Read the model definition and answer for the solid it produces. Units are mm, in the model's axes. Face numbers are marked on the shaded views. A direction names the side the tool comes from. Coordinates: 2 decimals unless noted, no trailing zeros. Loops run counter-clockwise (first coordinate to the right, second up) from the corner with the lowest first, then second, coordinate; pieces in that order, holes last. Notation, with made-up numbers: (38.25, 1.5) - (74.25, 1.5) arc R13 cw to (74.25, 13.5) - close; hole circle Ø7 at (-28.5, 2). An arc over 180 degrees is marked (long way). Use one line per item in the form item = value.
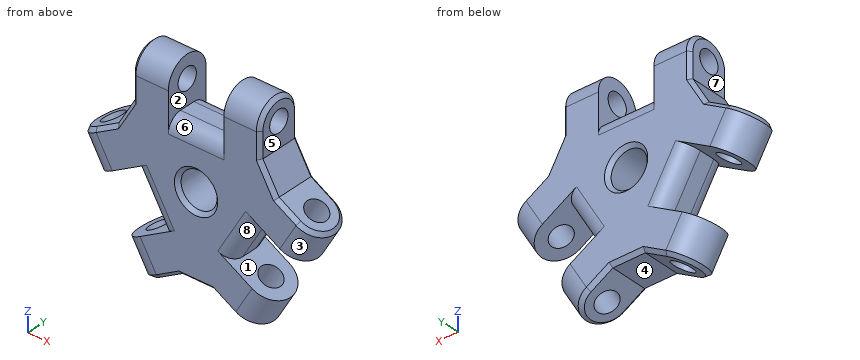
from build123d import *

# Parameters (mm, degrees)
SKETCH1_R           = 2.5
BOSS_EXTRUDE1_DEPTH = 3.1
CUT_EXTRUDE1_START  = -26.968876556
SKETCH2_R           = 1.5
CUT_EXTRUDE1_DEPTH  = 36.237753113
CIRPATTERN5_COUNT   = 3
FILLET2_R           = 2
CHAMFER1_SIZE       = 0.5


with BuildPart() as part:
    # Sketch1 → Boss-Extrude1 (new body, symmetric)
    with BuildSketch(Plane(origin=(0, 0, 0), x_dir=(1, 0, 0), z_dir=(0, 1, 0))):
        Polygon((-8.85, -7.707626094), (-8.85, -14.657626094), (-3.85, -14.657626094), (-3.85, -7.707626094), (3.85, -7.707626094), (3.85, -14.657626094), (8.85, -14.657626094), (8.85, -7.707626094), (11.1, -3.810511777), (17.118876556, -0.335511777), (14.618876556, 3.994615242), (8.6, 0.519615242), (4.75, 7.188010851), (10.768876556, 10.663010851), (8.268876556, 14.99313787), (2.25, 11.51813787), (-2.25, 11.51813787), (-8.268876556, 14.99313787), (-10.768876556, 10.663010851), (-4.75, 7.188010851), (-8.6, 0.519615242), (-14.618876556, 3.994615242), (-17.118876556, -0.335511777), (-11.1, -3.810511777), align=None)
        Circle(SKETCH1_R, mode=Mode.SUBTRACT)
    extrude(amount=BOSS_EXTRUDE1_DEPTH, both=True)

    # Sketch2 → Cut-Extrude1 (cut)
    with BuildSketch(Plane.ZY.offset(8.85).offset(CUT_EXTRUDE1_START)):
        with Locations((11.182626094, 0)):
            Circle(SKETCH2_R)
        with BuildLine():
            Line((11.182626094, 3.1), (14.657626094, 3.1))
            Line((14.657626094, 3.1), (14.657626094, -3.1))
            Line((14.657626094, -3.1), (11.182626094, -3.1))
            ThreePointArc((11.182626094, -3.1), (14.282626094, 0), (11.182626094, 3.1))
        make_face()
    cut_extrude1 = extrude(amount=CUT_EXTRUDE1_DEPTH, mode=Mode.SUBTRACT)

    # CirPattern5: Cut-Extrude1 ×3 about axis
    cirpattern5_axis = Axis((0, 3.1, 0), (0, -1, 0))
    for i in range(1, CIRPATTERN5_COUNT):
        add(cut_extrude1.rotate(cirpattern5_axis, i * 360 / CIRPATTERN5_COUNT), mode=Mode.SUBTRACT)

    # Fillet2
    fillet2_edges = [part.edges().sort_by_distance(p)[0] for p in [
        (6.675, 3.1, -3.853813047),
        (0, -3.1, 7.707626094),
        (-6.675, -3.1, -3.853813047),
        (6.675, -3.1, -3.853813047),
        (-6.675, 3.1, -3.853813047),
        (0, 3.1, 7.707626094),
    ]]
    fillet(fillet2_edges, radius=FILLET2_R)

    # Chamfer1
    chamfer1_edges = [part.edges().sort_by_distance(p)[0] for p in [
        (-12.604719139, -3.1, 2.941761777),
        (-12.604719139, 3.1, 2.941761777),
        (-16.79411703, 0, 0.523011777),
        (3.754719139, -3.1, -12.38688787),
        (3.754719139, 3.1, -12.38688787),
        (7.94411703, 0, -14.80563787),
        (16.79411703, 0, 0.523011777),
        (-7.94411703, 0, -14.80563787),
        (-8.85, -3.1, 9.445126094),
        (-9.975, -3.1, 5.759068935),
        (-3.754719139, -3.1, -12.38688787),
        (0, -3.1, -11.51813787),
        (12.604719139, -3.1, 2.941761777),
        (9.975, -3.1, 5.759068935),
        (0, 3.1, -11.51813787),
        (-3.754719139, 3.1, -12.38688787),
        (9.975, 3.1, 5.759068935),
        (-2.5, -3.1, 0),
        (-2.5, 3.1, 0),
        (-9.975, 3.1, 5.759068935),
        (8.85, -3.1, 9.445126094),
        (-8.85, 3.1, 9.445126094),
        (8.85, 3.1, 9.445126094),
        (8.85, 0, 14.282626094),
        (-8.85, 0, 14.282626094),
        (12.604719139, 3.1, 2.941761777),
    ]]
    chamfer(chamfer1_edges, length=CHAMFER1_SIZE)


solid = part.part
Item 1: Find the intervals of material crossed by L1, parallel to X at y = 0, z = -2.25; L2, parallel to X at y = 0, z = 13; L3, parallel to X at y = -0.5, z = -10.5, in increasing order.
Results below:
L1 = -15.19 to -13.35, -7.6 to -1.09, 1.09 to 7.6, 13.35 to 15.19
L2 = -8.85 to -3.85, 3.85 to 8.85
L3 = -10.38 to -8.48, -5.22 to 5.22, 8.48 to 10.38
Item 2: The part is cut by section B-B on y = -0.5. Count the separate pieces of the cut face and the enclosed holes in it, plus the area to 3 significant figures.
Results below:
separate_pieces = 7
enclosed_holes = 1
area = 373 mm²
Item 3: For a pull along Z with two mould halves and no side action, classify the marked faces 1, 2 and 3 as +Z half, -Z half, draft (parallel to the pull), parting line (faces both ways), or undercut.
Results below:
face_1 = undercut
face_2 = draft
face_3 = -Z half
Item 4: Which of the six approach directions +Z, -Z, +X, -X, +Y, -Y give full straight-line access (tool end or side, diameter ignored) to the marked faces 4, 5, 6, 7 and 8?
Results below:
face_4 = -Z, +Y, -Y
face_5 = +Z, +X, +Y, -Y
face_6 = +Z, -Y
face_7 = +Z, -X, +Y, -Y
face_8 = -Y
Item 5: Each of these flat-tipped pins is pushed along its axis until it touches: P1, Ø2, axis at x = 12.5, y = -2, coming from the -Z side; P2, Ø2, axis at y = 1, z = -3, coming from the -X side; P3, Ø0.7, axis at x = -1.5, y = 0, coming from the +Z side. Where does it stop, or does it pass through?
Results below:
P1 = -3.35
P2 = -15.22
P3 = 7.71
Item 6: The part is cut by section A-A on x = 0. Give the vertices of the cut face in (y, z), plus the area to 3 significant figures.
Results below:
outline = (-3.1, -11.02) - (-2.6, -11.52) - (2.6, -11.52) - (3.1, -11.02) - (3.1, -3) - (2.6, -2.5) - (-2.6, -2.5) - (-3.1, -3) - close; (-3.1, 3) - (-2.6, 2.5) - (2.6, 2.5) - (3.1, 3) - (3.1, 5.71) arc R2 ccw to (1.1, 7.71) - (-1.1, 7.71) arc R2 ccw to (-3.1, 5.71) - close
area = 85.7 mm²
